Check sheet for the modelled part. Datum: model origin and axes. Units: mm. Round coordinates to 2 decimals unless told otherwise and drop trailing zeros. Write each loop counter-clockwise with the first axis right and the second up, starting at its lowest first coordinate (ties: lowest second). Pieces come first, ordered by that corner, then holes. Notation, with made-up numbers: (47.5, -33.5) -> (67.5, -33.5) arc R14 cw to (67.5, -29.5) -> close; hole circle Ø5 at (5.25, 32). An arc over 180 degrees is marked (long way). Answer as a JSON object with one key per item and string values. Group by question number.
```python
from build123d import *

# Parameters (mm, degrees)
SKETCH1_R           = 1
BOSS_EXTRUDE1_DEPTH = 0.7
SKETCH2_W           = 25.502878438
SKETCH2_H           = 1.8
CUT_EXTRUDE1_DEPTH  = 10
BOSS_EXTRUDE2_DEPTH = 0.7
SKETCH6_W           = 5.25
SKETCH6_H           = 9.55
CUT_EXTRUDE2_DEPTH  = 6


with BuildPart() as part:
    # Sketch1 → Boss-Extrude1 (new body)
    with BuildSketch(Plane(origin=(0, 0, 0), x_dir=(1, 0, 0), z_dir=(0, 1, 0))):
        Polygon((20.240139403, -28.5), (20.75, -27.990139403), (20.75, 27.990139403), (20.240139403, 28.5), (-20.240139403, 28.5), (-20.75, 27.990139403), (-20.75, -27.990139403), (-20.240139403, -28.5), align=None)
        with Locations((-19, -27)):
            Circle(SKETCH1_R, mode=Mode.SUBTRACT)
        with Locations((19, -27)):
            Circle(SKETCH1_R, mode=Mode.SUBTRACT)
        with Locations((-9.45, 2.115469811)):
            Circle(SKETCH1_R, mode=Mode.SUBTRACT)
        with Locations((-9.45, 6.284530189)):
            Circle(SKETCH1_R, mode=Mode.SUBTRACT)
        with Locations((-19, 27)):
            Circle(SKETCH1_R, mode=Mode.SUBTRACT)
        with Locations((19, 27)):
            Circle(SKETCH1_R, mode=Mode.SUBTRACT)
    extrude(amount=BOSS_EXTRUDE1_DEPTH)

    # Sketch2 → Cut-Extrude1 (cut)
    with BuildSketch(Plane(origin=(0, 0.7, 0), x_dir=(1, 0, 0), z_dir=(0, 1, 0))):
        with Locations((7.248560781, -22)):
            Rectangle(SKETCH2_W, SKETCH2_H)
    extrude(amount=-CUT_EXTRUDE1_DEPTH, mode=Mode.SUBTRACT)

    # Sketch5 → Boss-Extrude2 (add)
    with BuildSketch(Plane(origin=(0, 0.7, 0), x_dir=(1, 0, 0), z_dir=(0, 1, 0))):
        Polygon((-19.540139403, -29.2), (19.540139403, -29.2), (20.240139403, -28.5), (-20.240139403, -28.5), align=None)
    extrude(amount=-BOSS_EXTRUDE2_DEPTH)

    # Sketch6 → Cut-Extrude2 (cut)
    with BuildSketch(Plane(origin=(0, 0.7, 0), x_dir=(1, 0, 0), z_dir=(0, 1, 0))):
        with Locations((-18.125, 17.048605705)):
            Rectangle(SKETCH6_W, SKETCH6_H)
    extrude(amount=-CUT_EXTRUDE2_DEPTH, mode=Mode.SUBTRACT)


solid = part.part
```
(1) Scan lines: line 1 along Z through (x, y) = (19, 0.45); line 2 along Z through (x, y) = (-19, 0.5); line 3 along X through (y, z) = (0.35, 27). Record each from-to range of solid material in increasing order.
(2) Section check C-C on x = -9.45. Record the cut outline in (y, z).
(3) Release check for a two-part mould opening along Z. For faces 1 (the flat face through (0, 0, 0)), 2 (the cylindrical face through (-20, 0.3, 27)), 3 (the flat face through (20.14, 0.35, 28.6)) record: pulls with the +Z half, pulls with the -Z half, needs draft (parallel to the pull), parting line crosses it, or undercut.
(4) Section check D-D on y = 0.4. Record the cut outline in (x, z).
(5) Section check B-B on z = -27. Record the cut outline in (x, y), then the cut area to 4 significant figures.
(6) Section check A-A on x = 2. Record the cut outline in (y, z).
Data:
{
 "1": {"line 1": "z = -28.5 to -28, -26 to 21.1, 22.9 to 26, 28 to 29.2", "line 2": "z = -28.5 to -28, -26 to -21.82, -12.27 to 26, 28 to 29.2", "line 3": "x = -20.75 to -20, -18 to 18, 20 to 20.75"},
 "2": {"outline": "(0, -28.5) -> (0.7, -28.5) -> (0.7, -7.28) -> (0, -7.28) -> close; (0, -5.28) -> (0.7, -5.28) -> (0.7, -3.12) -> (0, -3.12) -> close; (0, -1.12) -> (0.7, -1.12) -> (0.7, 29.2) -> (0, 29.2) -> close"},
 "3": {"face 1": "needs draft", "face 2": "undercut", "face 3": "pulls with the +Z half"},
 "4": {"outline": "(-20.75, -27.99) -> (-20.24, -28.5) -> (20.24, -28.5) -> (20.75, -27.99) -> (20.75, 27.99) -> (19.54, 29.2) -> (-19.54, 29.2) -> (-20.75, 27.99) -> (-20.75, -12.27) -> (-15.5, -12.27) -> (-15.5, -21.82) -> (-20.75, -21.82) -> close; hole circle Ø2 at (-19, -27); hole circle Ø2 at (-19, 27); hole circle Ø2 at (-9.45, -6.28); hole circle Ø2 at (-9.45, -2.12); hole (-5.5, 21.1) -> (20, 21.1) -> (20, 22.9) -> (-5.5, 22.9) -> close; hole circle Ø2 at (19, -27); hole circle Ø2 at (19, 27)"},
 "5": {"outline": "(-20.75, 0) -> (-20, 0) -> (-20, 0.7) -> (-20.75, 0.7) -> close; (-18, 0) -> (18, 0) -> (18, 0.7) -> (-18, 0.7) -> close; (20, 0) -> (20.75, 0) -> (20.75, 0.7) -> (20, 0.7) -> close", "area": "26.25 mm²"},
 "6": {"outline": "(0, -28.5) -> (0.7, -28.5) -> (0.7, 21.1) -> (0, 21.1) -> close; (0, 22.9) -> (0.7, 22.9) -> (0.7, 29.2) -> (0, 29.2) -> close"}
}
